Answer from the drawing. Dimensions are ordinates in mm from the lowest x, y and z of the part. A direction names the side the tool comes from. Coordinates: 2 decimals unless noted, no trailing zeros. Order: outer loops, then holes, each group sorted by start corner. A loop starts at its lowest first (then second) coordinate and runs counter-clockwise, first axis right, second up. Notation, with made-up numbers: (72, 57) - (90, 57) arc R16 cw to (90, 67) - close; hole circle Ø4 at (38, 4). An arc over 180 degrees is marked (long way). Answer as a JSON object with one key per item and string values. Group by question number.
1) Each of these flat-tipped pins is pushed along its axis until it touches: P1, Ø3, axis at y = 22, z = 8.5, coming from the +X side; P2, Ø1.3, axis at x = 6, z = 8.5, coming from the +Y side; P3, Ø4, axis at x = 11, y = 22, coming from the -Z side. Where does it stop, or does it pass through?
2) Section A-A (z = 7.5) is taken. Give the vertices of the cut face in (x, y), plus the area to 4 significant figures.
3) Section D-D (x = 3) is taken. Give the vertices of the cut face in (y, z).
4) Section B-B (x = 6.5) is taken. Give the vertices of the cut face in (y, z), plus the area to 4 significant figures.
5) Find the intervals of material crossed by line 1 along X through (y, z) = (26.25, 7.5); line 2 along Z through (x, y) = (6.5, 25.8); line 3 along Y through (x, z) = (5, 13.5), in increasing order.
6) Section C-C (y = 24.5) is taken. Give the vertices of the cut face in (x, z), plus the area to 4 significant figures.
7) A tool of negligible diameter and unlimited length cuts with its end or side. For the marked faces 1, 2 and 3, from which of +Z, -Z, +X, -X, +Y, -Y can it reach the whole face along a straight path? Write none if from no direction.
8) The mould has two halves that part along Z. Classify the marked faces 4, 5, 6 and 7: released by +Z, released by -Z, zero draft, split by the parting line, or undercut.
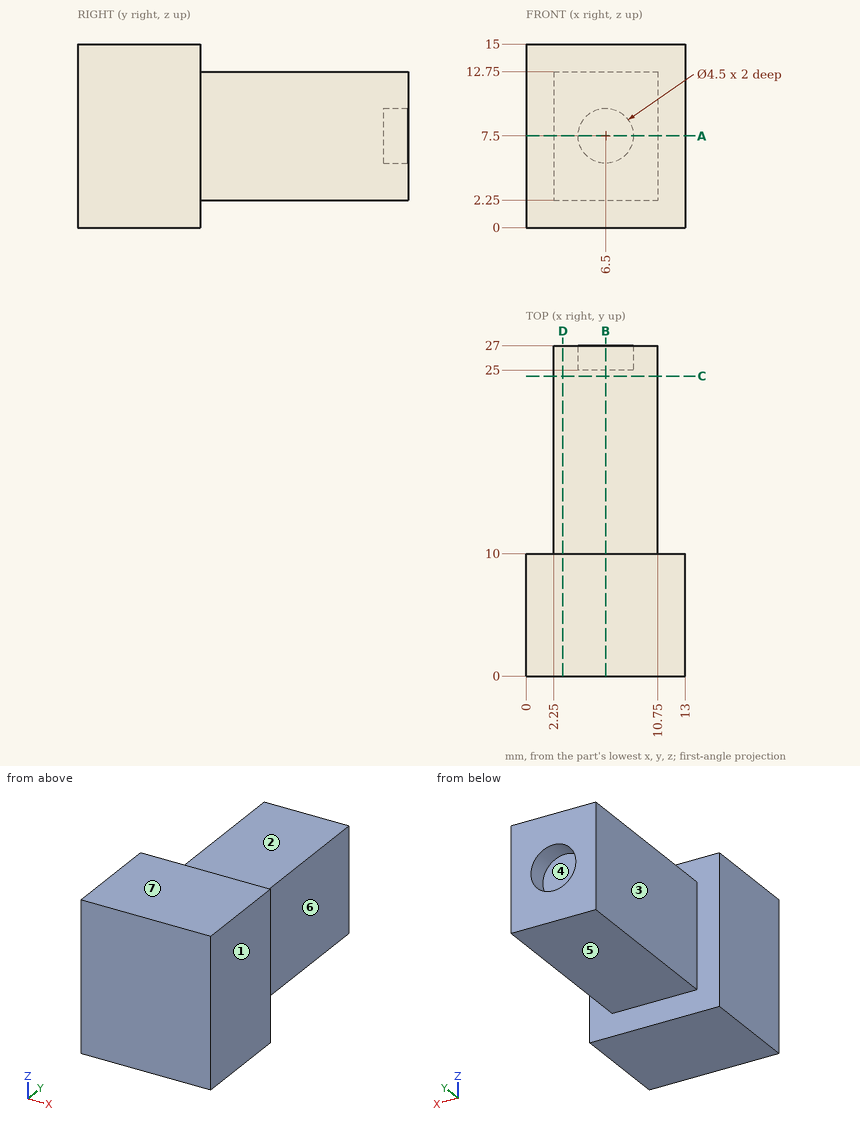
Report:
{
 "1": {"P1": "stops at x = 10.75", "P2": "stops at y = 25", "P3": "stops at z = 2.25"},
 "2": {"outline": "(0, 0) - (13, 0) - (13, 10) - (10.75, 10) - (10.75, 27) - (8.75, 27) - (8.75, 25) - (4.25, 25) - (4.25, 27) - (2.25, 27) - (2.25, 10) - (0, 10) - close", "area": "265.5 mm²"},
 "3": {"outline": "(0, 0) - (10, 0) - (10, 2.25) - (27, 2.25) - (27, 12.75) - (10, 12.75) - (10, 15) - (0, 15) - close"},
 "4": {"outline": "(0, 0) - (10, 0) - (10, 2.25) - (27, 2.25) - (27, 5.25) - (25, 5.25) - (25, 9.75) - (27, 9.75) - (27, 12.75) - (10, 12.75) - (10, 15) - (0, 15) - close", "area": "319.5 mm²"},
 "5": {"line 1": "x = 2.25 to 4.25, 8.75 to 10.75", "line 2": "z = 2.25 to 5.25, 9.75 to 12.75", "line 3": "y = 0 to 10"},
 "6": {"outline": "(2.25, 2.25) - (10.75, 2.25) - (10.75, 12.75) - (2.25, 12.75) - close", "area": "89.25 mm²"},
 "7": {"face 1": "+Z, -Z, +X, +Y, -Y", "face 2": "+Z, +X, -X, +Y", "face 3": "+Z, -Z, -X, +Y"},
 "8": {"face 4": "undercut", "face 5": "released by -Z", "face 6": "zero draft", "face 7": "released by +Z"}
}
